```python
from build123d import *

# Parameters (mm, degrees)
PAD008_DEPTH       = 36
SKETCH008_W        = 24
SKETCH008_H        = 56
POCKET_DEPTH       = 59.001
SKETCH009_W        = 60
SKETCH009_H        = 48
POCKET001_DEPTH    = 51
SKETCH010_R        = 12
SKETCH010_R_2      = 1.75
POCKET002_DEPTH    = 5
SKETCH011_R        = 5
PAD009_DEPTH       = 4
SKETCH012_R        = 2.4
POCKET003_DEPTH    = 8
SKETCH015_R        = 1.5
POCKET005_DEPTH    = 10
SKETCH022_R        = 1.1
POCKET006007_DEPTH = 10
SKETCH026_R        = 1.4
POCKET006008_DEPTH = 72.001
SKETCH027_W        = 31.606602
SKETCH027_H        = 56
POCKET006009_DEPTH = 52


with BuildPart() as part:
    # Sketch007 → Pad008 (new body, symmetric)
    with BuildSketch(Plane.YZ):
        Polygon((9.606602, -1), (0, -10.606602), (-9.606602, -1), (-19.606602, -1), (-19.606602, -60), (94.606602, -60), (94.606602, -1), (84.606602, -1), (75, -10.606602), (65.393398, -1), align=None)
    extrude(amount=PAD008_DEPTH, both=True)

    # Sketch008 → Pocket (cut, through all)
    with BuildSketch(Plane(origin=(0, 0, -1), x_dir=(0, -1, 0), z_dir=(0, 0, 1))):
        with Locations((-32, 0)):
            Rectangle(SKETCH008_W, SKETCH008_H)
    extrude(amount=-POCKET_DEPTH, mode=Mode.SUBTRACT)

    # Sketch009 → Pocket001 (cut)
    with BuildSketch(Plane.YX.offset(60)):
        with Locations((79, 0)):
            Rectangle(SKETCH009_W, SKETCH009_H)
    extrude(amount=-POCKET001_DEPTH, mode=Mode.SUBTRACT)

    # Sketch010 → Pocket002 (cut)
    with BuildSketch(Plane(origin=(0, 44, 0), x_dir=(0, 0, -1), z_dir=(0, -1, 0))):
        with Locations((32, 0)):
            Circle(SKETCH010_R)
        with Locations((16.5, 15.5)):
            Circle(SKETCH010_R_2)
        with Locations((47.5, 15.5)):
            Circle(SKETCH010_R_2)
        with Locations((47.5, -15.5)):
            Circle(SKETCH010_R_2)
        with Locations((16.5, -15.5)):
            Circle(SKETCH010_R_2)
    extrude(amount=-POCKET002_DEPTH, mode=Mode.SUBTRACT)

    # Sketch011 → Pad009 (new body)
    with BuildSketch(Plane(origin=(0, 44, 0), x_dir=(0, 0, -1), z_dir=(0, -1, 0))):
        with Locations((8, 11)):
            Circle(SKETCH011_R)
        with Locations((8, -11)):
            Circle(SKETCH011_R)
    extrude(amount=PAD009_DEPTH)

    # Sketch012 → Pocket003 (cut)
    with BuildSketch(Plane(origin=(0, 40, 0), x_dir=(0, 0, -1), z_dir=(0, -1, 0))):
        with Locations((8, 11)):
            Circle(SKETCH012_R)
        with Locations((8, -11)):
            Circle(SKETCH012_R)
    extrude(amount=-POCKET003_DEPTH, mode=Mode.SUBTRACT)

    # Sketch015 → Pocket005 (cut)
    with BuildSketch(Plane(origin=(0, 0, -1), x_dir=(0, -1, 0), z_dir=(0, 0, 1))):
        with Locations((-89.606602, 30)):
            Circle(SKETCH015_R)
        with Locations((-89.606602, 18)):
            Circle(SKETCH015_R)
        with Locations((-60.393398, 30)):
            Circle(SKETCH015_R)
        with Locations((-60.393398, 18)):
            Circle(SKETCH015_R)
        with Locations((-89.606602, -18)):
            Circle(SKETCH015_R)
        with Locations((-89.606602, -30)):
            Circle(SKETCH015_R)
        with Locations((-60.393398, -18)):
            Circle(SKETCH015_R)
        with Locations((-60.393398, -30)):
            Circle(SKETCH015_R)
        with Locations((-14.606602, 30)):
            Circle(SKETCH015_R)
        with Locations((14.606602, 18)):
            Circle(SKETCH015_R)
        with Locations((14.606602, 30)):
            Circle(SKETCH015_R)
        with Locations((-14.606602, 18)):
            Circle(SKETCH015_R)
        with Locations((-14.606602, -18)):
            Circle(SKETCH015_R)
        with Locations((-14.606602, -30)):
            Circle(SKETCH015_R)
        with Locations((14.606602, -18)):
            Circle(SKETCH015_R)
        with Locations((14.606602, -30)):
            Circle(SKETCH015_R)
    extrude(amount=-POCKET005_DEPTH, mode=Mode.SUBTRACT)

    # Sketch022 → Pocket006007 (cut)
    with BuildSketch(Plane.ZX.offset(94.606602)):
        with Locations((-15.75, -26.5)):
            Circle(SKETCH022_R)
        with Locations((-6.25, -26.5)):
            Circle(SKETCH022_R)
    extrude(amount=-POCKET006007_DEPTH, mode=Mode.SUBTRACT)

    # Sketch026 → Pocket006008 (cut, through all)
    with BuildSketch(Plane(origin=(-36, 0, 0), x_dir=(0, 1, 0), z_dir=(-1, 0, 0))):
        with Locations((30, 45)):
            Circle(SKETCH026_R)
        with Locations((43, 45)):
            Circle(SKETCH026_R)
        with Locations((43, 21)):
            Circle(SKETCH026_R)
        Polygon((8, 13), (27, 32), (8, 51), (-11, 32), align=None)
        Polygon((72, 13), (91, 32), (72, 51), (53, 32), align=None)
    extrude(amount=-POCKET006008_DEPTH, mode=Mode.SUBTRACT)

    # Sketch027 → Pocket006009 (cut)
    with BuildSketch(Plane.YX.offset(60)):
        with Locations((4.196699, 0)):
            Rectangle(SKETCH027_W, SKETCH027_H)
    extrude(amount=-POCKET006009_DEPTH, mode=Mode.SUBTRACT)


solid = part.part
```
Source: CAD feature listing. Evaluate the final solid. Frame: model axes, mm. A direction names the side the tool comes from. Coordinates: 2 decimals unless noted, no trailing zeros. Write each loop counter-clockwise with the first axis right and the second up, starting at its lowest first coordinate (ties: lowest second). Pieces come first, ordered by that corner, then holes. Notation, with made-up numbers: (51.5, -36) -> (65.5, -36) arc R9 ccw to (65.5, -21) -> close; hole circle Ø1 at (-31, 22.5). An arc over 180 degrees is marked (long way). Return JSON: item names as keys, results as strings. Group by question number.
1) Section query B-B, the plane z = -34.5. State how many separate pieces and enclosed holes the cut face has, plus the area to 3 significant figures.
2) Section query A-A, the plane y = 30. Return loops of the section in (x, z), plus the area to 3 significant figures.
3) Mould query, pull axis Y, two halves, no side actions, for faces 1 (the face through (-24, 61, -41)), 2 (the face through (-30, 60, -11)). Classes: +Y half, -Y half, draft (parallel to the pull), parting line (faces both ways), or undercut.
4) Set-up query: faces 3 (the face through (-8.7, 40, -6.8)), 4 (the face through (-28.735, 59.587, -5.93)), 5 (the face through (-32, 18, -41)). Return all of +Z, -Z, +X, -X, +Y, -Y with unobstructed straight access to the full face (end or side cutting, diameter ignored); none if empty.
5) Contact query for flat-ended pins moving along their axis: P1, Ø1.5, axis at x = -3, y = 18.5, coming from the -Z side; P2, Ø2.5, axis at x = 30, y = 14.61, coming from the +Z side; P3, Ø10, axis at x = -5.5, y = 37.5, coming from the +Z side. Output: stop coordinate, or through.
6) Ray query, line 1 along X through (y, z) = (31.5, -48.5); line 2 along X through (y, z) = (89.75, -15.75); line 3 along X through (y, z) = (74, -50). Return the intervals inside material, ascending.
From the geometry:
{
 "1": {"separate pieces": "5", "enclosed holes": "0", "area": "1,480 mm²"},
 "2": {"outline": "(-36, -60) -> (-28, -60) -> (-28, -46.4) -> (-36, -46.4) -> close; (-36, -43.6) -> (-28, -43.6) -> (-28, -1) -> (-36, -1) -> close; (28, -60) -> (36, -60) -> (36, -46.4) -> (28, -46.4) -> close; (28, -43.6) -> (36, -43.6) -> (36, -1) -> (28, -1) -> close", "area": "899 mm²"},
 "3": {"face 1": "draft", "face 2": "undercut"},
 "4": {"face 3": "+Z, -Z", "face 4": "+Z", "face 5": "+X, -X"},
 "5": {"P1": "z = -8", "P2": "z = -11", "P3": "z = -3.14"},
 "6": {"line 1": "-36 to -28, 28 to 36", "line 2": "-36 to -27.6, -25.4 to -24, 24 to 36", "line 3": "-36 to -24, 24 to 36"}
}
